Can you work these out from the drawing? Everything is in mm from the part's minimum corner. A direction names the side the tool comes from. Round coordinates to 2 decimals unless told otherwise and drop trailing zeros. Order: outer loops, then holes, each group sorted by start corner. A loop starts at its lowest first (then second) coordinate and runs counter-clockwise, first axis right, second up. Notation, with made-up numbers: M -25.75,60 L -1.75,60 A4 ccw -1.75,64 Z; hole C 74,63 d8. An arc over 180 degrees is marked long. Write each question's results on one line, items separated by ' | '. Start each with the question number.
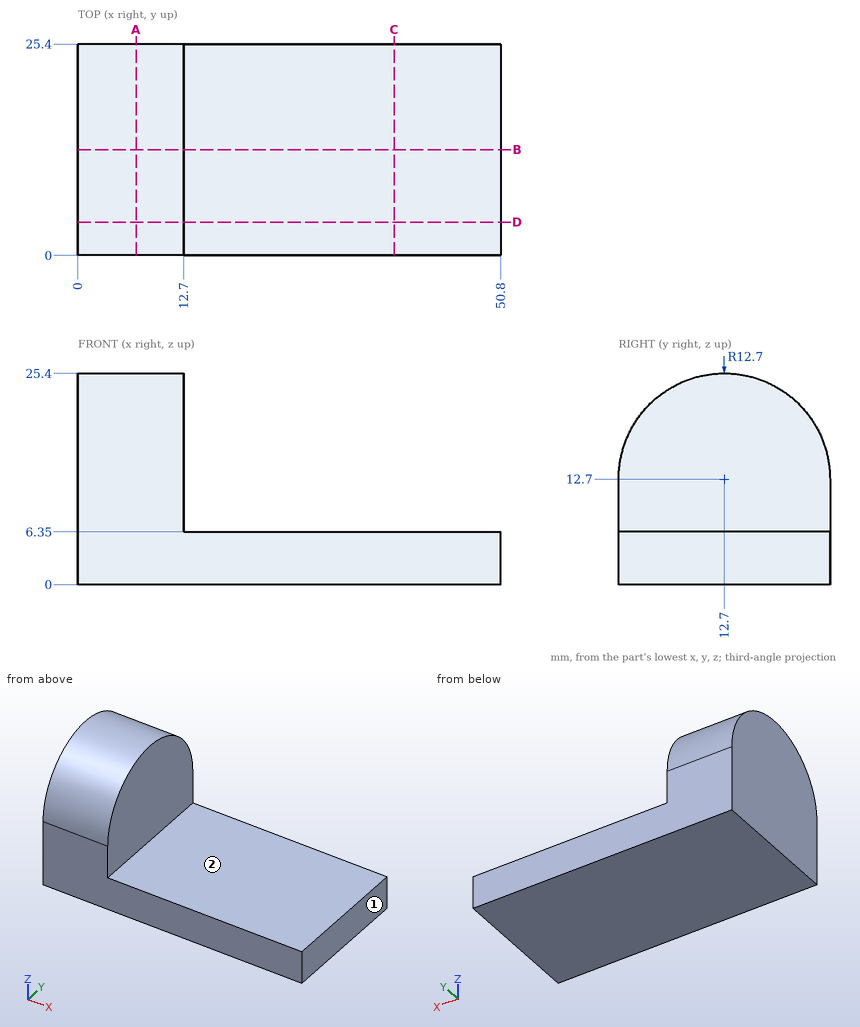
(1) I want a section at B-B on y = 12.7. Write out the boundary of the cut face in (x, z), and give its area (3 significant figures).
(2) On a 3-axis mill with a long thin cutter (end or side, diameter ignored), from which of +Z, -Z, +X, -X, +Y, -Y can I reach the whole of each face in a straight line? I mean the marked faces 1 and 2. Say none if no direction works.
(3) I'm going to push flat-ended pins straight in: pin 1 Ø5 at (x, y) = (22, 7) entering from -Z; pin 2 Ø2 at (x, y) = (33.5, 10.5) entering from +Z; pin 3 Ø2 at (y, z) = (18.5, 13.5) entering from +X. Where does each tip first touch, or does it pass through?
(4) I want a section at A-A on x = 7. Write out the boundary of the cut face in (y, z), and give its area (3 significant figures).
(5) Please list where these lines run through material, in increasing order: line 1 (Z direction, x = 32.5, y = 8); line 2 (X direction, y = 13, z = 17); line 3 (Y direction, x = 12.5, z = 22).
(6) I want a section at D-D on y = 4. Write out the boundary of the cut face in (x, z), and give its area (3 significant figures).
(7) I want a section at C-C on x = 38. Write out the boundary of the cut face in (y, z), and give its area (3 significant figures).
Solutions:
1) outline: M 0,0 L 50.8,0 L 50.8,6.35 L 12.7,6.35 L 12.7,25.4 L 0,25.4 Z | area: 565 mm^2
2) face 1: +Z, -Z, +X, +Y, -Y | face 2: +Z, +X, +Y, -Y
3) pin 1: z = 0 | pin 2: z = 6.35 | pin 3: x = 12.7
4) outline: M 0,0 L 25.4,0 L 25.4,12.7 A12.7 ccw 0,12.7 Z | area: 576 mm^2
5) line 1: 0 to 6.35 | line 2: 0 to 12.7 | line 3: 4.05 to 21.35
6) outline: M 0,0 L 50.8,0 L 50.8,6.35 L 12.7,6.35 L 12.7,21.95 L 0,21.95 Z | area: 521 mm^2
7) outline: M 0,0 L 25.4,0 L 25.4,6.35 L 0,6.35 Z | area: 161 mm^2
